Verification items for the finished model (mm, model axes). A direction names the side the tool comes from. Round coordinates to 2 decimals unless told otherwise and drop trailing zeros. Order: outer loops, then holes, each group sorted by start corner. A loop starts at its lowest first (then second) coordinate and runs counter-clockwise, first axis right, second up. Notation, with made-up numbers: M 13,59 L 43,59 A24 cw 43,94 Z; hole C -17,53 d5. An arc over 180 degrees is marked long. Use one line per item in the form item = value. Start each with the question number.
Item 1: Tool access check on faces 4 (the flat face through (13, -10, 10)), 5 (the cylindrical face through (-14.985, 0.66, 4.437)). Record the directions out of +Z, -Z, +X, -X, +Y, -Y that give a thin tool (end or side, any length) a straight path to the whole face; none if there is none.
Item 2: Release check for a two-part mould opening along X. For faces 1 (the flat face through (0, 0, -3)), 2 (the cylindrical face through (-2.343, 17.847, 3.577)), 3 (the flat face through (0, 0, 0)) record: +X half, -X half, draft (parallel to the pull), parting line (faces both ways), or undercut.
Item 3: Cross-section at A-A on y = 0. Enter the section's corners in (x, z).
Item 4: Cross-section at C-C on z = 5.75. Enter the section's corners in (x, y).
Item 5: Go/stop test with flat-tipped pins: pin 1 Ø4 at (x, z) = (-8, 8) entering from +Y; pin 2 Ø6 at (y, z) = (12, 2) entering from -X; pin 3 Ø1.5 at (x, y) = (4.5, 4) entering from +Z. Record where each tip stops, or that it passes through.
Item 6: Thickness scan on probe 1 along Y at (x, z) = (0, 5); probe 2 along Z at (x, y) = (-2.5, -9.5); probe 3 along X at (y, z) = (8.5, 4.25). Record the ranges inside material, lowest first. Write a range as [from, to].
Item 7: Cross-section at D-D on z = -1. Enter the section's corners in (x, y), then the cut area to 3 significant figures.
from build123d import *

# Parameters (mm, degrees)
F0_R     = 18
F0_R_2   = 15
F1_DEPTH = 10
F2_R     = 18
F3_DEPTH = 3
F4_R     = 1


with BuildPart() as f1:
    # F0 (on Top) → F1 (new body)
    with BuildSketch(Plane.XY):
        Circle(F0_R)
        Circle(F0_R_2, mode=Mode.SUBTRACT)
    extrude(amount=F1_DEPTH)

    # F2 (on face) → F3 (join)
    with BuildSketch(Plane.XY):
        Circle(F2_R)
    extrude(amount=-F3_DEPTH)

    # F4
    f4_edges = [f1.edges().sort_by_distance(p)[0] for p in [
        (-18, 0, 10),
        (-15, 0, 10),
        (-18, 0, -3),
    ]]
    fillet(f4_edges, radius=F4_R)


solid = f1.part
Output values:
q1.face_4 = +Z, +X, -X, +Y, -Y
q1.face_5 = +Z
q2.face_1 = draft
q2.face_2 = parting line
q2.face_3 = undercut
q3.outline = M -18,-2 A1 ccw -17,-3 L 17,-3 A1 ccw 18,-2 L 18,9 A1 ccw 17,10 L 16,10 A1 ccw 15,9 L 15,0 L -15,0 L -15,9 A1 ccw -16,10 L -17,10 A1 ccw -18,9 Z
q4.outline = C 0,0 d36; hole C 0,0 d30
q5.pin_1 = 16.97
q5.pin_2 = -15.59
q5.pin_3 = 0
q6.probe_1 = [-18, -15], [15, 18]
q6.probe_2 = [-3, 0]
q6.probe_3 = [-15.87, -12.36], [12.36, 15.87]
q7.outline = C 0,0 d36
q7.area = 1,020 mm2
